from build123d import *

# Parameters (mm, degrees)
F0_R     = 14.2875
F0_R_2   = 10.16
F1_DEPTH = 25.4
F2_DEPTH = 40.2336
F3_R     = 5.08


with BuildPart() as f1:
    # F0 (on Front) → F1 (new body)
    with BuildSketch(Plane.XZ):
        with BuildLine():
            ThreePointArc((5.042647, -28.126541), (21.916025, -18.336262), (28.575, 0))
            ThreePointArc((28.575, 0), (21.916025, 18.336262), (5.042647, 28.126541))
            ThreePointArc((5.042647, 28.126541), (-28.575, 0), (5.042647, -28.126541))
        make_face()
        Circle(F0_R, mode=Mode.SUBTRACT)
        with BuildLine():
            ThreePointArc((5.042647, 28.126541), (21.916025, 18.336262), (28.575, 0))
            ThreePointArc((28.575, 0), (21.916025, -18.336262), (5.042647, -28.126541))
            Line((5.042647, -28.126541), (57.336765, -18.751028))
            ThreePointArc((57.336765, -18.751028), (34.925, 0), (57.336765, 18.751028))
            Line((57.336765, 18.751028), (5.042647, 28.126541))
        make_face()
        with BuildLine():
            ThreePointArc((73.025, 0), (68.585683, 12.224174), (57.336765, 18.751028))
            ThreePointArc((57.336765, 18.751028), (34.925, 0), (57.336765, -18.751028))
            ThreePointArc((57.336765, -18.751028), (68.585683, -12.224174), (73.025, 0))
        make_face()
        with Locations((53.975, 0)):
            Circle(F0_R_2, mode=Mode.SUBTRACT)
    extrude(amount=F1_DEPTH)

    # F0 (on Front) → F2 (join)
    with BuildSketch(Plane.XZ):
        with BuildLine():
            ThreePointArc((5.042647, -28.126541), (21.916025, -18.336262), (28.575, 0))
            ThreePointArc((28.575, 0), (21.916025, 18.336262), (5.042647, 28.126541))
            ThreePointArc((5.042647, 28.126541), (-28.575, 0), (5.042647, -28.126541))
        make_face()
        Circle(F0_R, mode=Mode.SUBTRACT)
    extrude(amount=-F2_DEPTH)

    # F3
    f3_edges = [f1.edges().sort_by_distance(p)[0] for p in [
        (-5.042647, 40.2336, 28.126541),
    ]]
    fillet(f3_edges, radius=F3_R)


solid = f1.part
Design review of the part built by this model. Coordinates are the model's own, in mm. Give positions to 0.01 mm unless a question says otherwise; leave off trailing zeros. Write each loop counter-clockwise with the first axis right and the second up, starting at its lowest first coordinate (ties: lowest second). Pieces come first, ordered by that corner, then holes. Notation, with made-up numbers: M 86,72 L 97,72 A31 cw 97,103 Z; hole C 20.5,48.5 d11. An arc over 180 degrees is marked long. Answer as a JSON object with one key per item and string values. Group by question number.
1) We need section D-D (x = 30). Give the boundary of the cut face in (y, z).
2) Mouldability with a two-part tool opening along X and no side actions: class faces 1 (the face through (-14.274, 7.876, 0.628)), 2 (the face through (31.556, -12.522, 23.373)), 3 (the face through (43.825, -12.522, 0.447)), 4 (the face through (22, -25.4, 0)) as released by +X, released by -X, zero draft, split by the parting line, or undercut.
3) For line 1 along X through (y, z) = (-20.5, 8.5); line 2 along X through (y, z) = (9, -11); line 3 along Y through (x, z) = (28.5, 17), list the stretches that pass through material, from the lowest coordinate up.
4) Clearance check with flat-ended pins moving along their axes: pin 1 Ø1.5 at (y, z) = (-5, 16) entering from +X; pin 2 Ø2 at (y, z) = (24.5, -9.5) entering from -X; pin 3 Ø4 at (y, z) = (31, -19.5) entering from -X. State where each tip first meets the part, or that it passes through.
5) We need section A-A (y = -4.5). Count the separate pieces of the cut face and the enclosed holes in it, and give its area (3 significant figures).
Answer key:
{
 "1": {"outline": "M -25.4,-23.65 L 0,-23.65 L 0,23.65 L -25.4,23.65 Z"},
 "2": {"face 1": "undercut", "face 2": "released by +X", "face 3": "undercut", "face 4": "zero draft"},
 "3": {"line 1": "x = -27.28 to -11.48, 11.48 to 48.41, 59.54 to 71.02", "line 2": "x = -26.37 to -9.12, 9.12 to 26.37", "line 3": "y = -25.4 to 0"},
 "4": {"pin 1": "stops at x = 65.39", "pin 2": "stops at x = -27.28", "pin 3": "stops at x = -22.59"},
 "5": {"separate pieces": "1", "enclosed holes": "2", "area": "3,500 mm²"}
}
